from build123d import *

# Parameters (mm, degrees)
CROQUIS1_R                 = 2.38135
CROQUIS1_R_2               = 1.5875
SALIENTE_EXTRUIR1_DEPTH    = 70
CORTAR_EXTRUIR1_DEPTH      = 3.38135
CORTAR_EXTRUIR1_DEPTH_BACK = 3.38135
CROQUIS3_R                 = 5
CROQUIS3_R_2               = 1.5875
SALIENTE_EXTRUIR2_DEPTH    = 25
CROQUIS4_R                 = 10
CROQUIS4_R_2               = 1.5875
SALIENTE_EXTRUIR3_DEPTH    = 50
CROQUIS5_R                 = 5
SALIENTE_EXTRUIR4_DEPTH    = 10


with BuildPart() as part:
    # Croquis1 → Saliente-Extruir1 (new body)
    with BuildSketch(Plane(origin=(0, 0, 0), x_dir=(1, 0, 0), z_dir=(0, 1, 0))):
        Circle(CROQUIS1_R)
        Circle(CROQUIS1_R_2, mode=Mode.SUBTRACT)
    extrude(amount=SALIENTE_EXTRUIR1_DEPTH)

    # Croquis2 → Cortar-Extruir1 (cut, two sides)
    with BuildSketch(Plane.XY) as cortar_extruir1_sk:
        Polygon((2.38135, 70), (-2.38135, 70), (-2.38135, 69.160207489), align=None)
    extrude(amount=CORTAR_EXTRUIR1_DEPTH, mode=Mode.SUBTRACT)
    extrude(cortar_extruir1_sk.sketch, amount=-CORTAR_EXTRUIR1_DEPTH_BACK, mode=Mode.SUBTRACT)

    # Croquis3 → Saliente-Extruir2 (add)
    with BuildSketch(Plane.XZ):
        Circle(CROQUIS3_R)
        Circle(CROQUIS3_R_2, mode=Mode.SUBTRACT)
    extrude(amount=SALIENTE_EXTRUIR2_DEPTH)

    # Croquis4 → Saliente-Extruir3 (add)
    with BuildSketch(Plane.XZ.offset(25)):
        Circle(CROQUIS4_R)
        Circle(CROQUIS4_R_2, mode=Mode.SUBTRACT)
    extrude(amount=SALIENTE_EXTRUIR3_DEPTH)

    # Croquis5 → Saliente-Extruir4 (add)
    with BuildSketch(Plane.XY):
        with Locations((0, -12.25)):
            Circle(CROQUIS5_R)
    extrude(amount=SALIENTE_EXTRUIR4_DEPTH)


solid = part.part
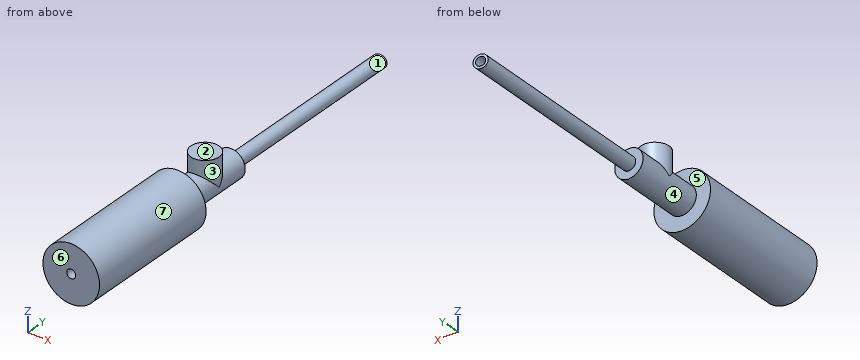
Build history of the part. All positions in model axes, mm. Face numbers are marked on the shaded views. A direction names the side the tool comes from. Give positions to 0.01 mm unless a question says otherwise; leave off trailing zeros. Order: outer loops, then holes, each group sorted by start corner. A loop starts at its lowest first (then second) coordinate and runs counter-clockwise, first axis right, second up. Notation, with made-up numbers: M -27,43.25 L 25,43.25 A24 ccw 25,53.25 Z; hole C 68,35 d2. An arc over 180 degrees is marked long. Use one line per item in the form item = value.
Q1. Wall check: probe 1 along Z at (x, y) = (0, 20); probe 2 along Z at (x, y) = (0, -20); probe 3 along Y at (x, z) = (-1, -5.5). Give the ranges that are in metal, low to high.
Conclusion:
probe_1 = -2.38 to -1.59, 1.59 to 2.38
probe_2 = -5 to -1.59, 1.59 to 5
probe_3 = -75 to -25
Q2. Slice it at A-A, the plane y = -12.25. Write the cut outline in (x, z) (1 decimal), and give its area (3 significant figures).
Conclusion:
outline = M -5,0 A5 ccw 5,0 L 5,10 L -5,10 Z; hole M -1.6,0 A1.6 ccw 1.6,0 Z
area = 135 mm2
Q3. Slice it at D-D, the plane y = 15.5. Write the cut outline in (x, z) (1 decimal), and give its area (3 significant figures).
Conclusion:
outline = C 0,0 d4.8; hole C 0,0 d3.2
area = 9.90 mm2
Q4. Slice it at C-C, the plane x = 6.75. Write the cut outline in (y, z), and give its area (3 significant figures).
Conclusion:
outline = M -75,-7.38 L -25,-7.38 L -25,7.38 L -75,7.38 Z
area = 738 mm2
Q5. Pull direction Y, two halves, no side cores. Call the marked faces 4, 5, 6 and 7: released by +Y, released by -Y, zero draft, split by the parting line, or undercut.
Conclusion:
face_4 = undercut
face_5 = undercut
face_6 = released by -Y
face_7 = zero draft
Q6. Slice it at B-B, the plane z = 8.25. Write the cut outline in (x, y).
Conclusion:
outline = M -5.65,-75 L 5.65,-75 L 5.65,-25 L -5.65,-25 Z; C 0,-12.25 d10
Q7. Which spindle directions (+Z, -Z, +X, -X, +Y, -Y) get a long thin tool onto all of the face, cutting with end or side? Do the marked faces 1, 2 and 3. Say none if no direction does.
Conclusion:
face_1 = +Y
face_2 = +Z, +X, -X, +Y, -Y
face_3 = +Z
Q8. Pin check, flat tips, straight feed: P1, Ø8, axis at x = -2, z = 7.5, coming from the +Y side; P2, Ø2, axis at x = 8, z = 4.5, coming from the +Y side; P3, Ø3, axis at y = -28.5, z = -1.5, coming from the -X side; P4, Ø6, axis at y = 44.5, z = -1.5, coming from the -X side. Stop position of each tip, or through.
Conclusion:
P1 = 0
P2 = -25
P3 = -10
P4 = -2.38
